Autodesk Inventor part; units mm, degrees
ref_plane "YZ Plane" through (0, 0, 0) normal (1, 0, 0) x (0, 1, 0)
ref_plane "XZ Plane" through (0, 0, 0) normal (0, 1, 0) x (-1, 0, 0)
ref_plane "XY Plane" through (0, 0, 0) normal (0, 0, 1) x (1, 0, 0)
sketch "Sketch1" plane through (0, 0, 0) normal (0, 1, 0) x (-1, 0, 0)
  line L0 (-15, 15) -> (15, 15)
  line L1 (15, 15) -> (15, -15)
  line L2 (15, -15) -> (-15, -15)
  line L3 (-15, -15) -> (-15, 15)
  line L4 (-15, 15) -> (15, -15) construction
  line L5 (15, 15) -> (-15, -15) construction
  circle A0 centre (0, 0) radius 3
  dimension "d0" = 30
  dimension "d1" = 30
  dimension "d2" = 6
extrude "Extrusion1" add sketch "Sketch1" along normal blind 35
The listing builds one solid part. Answer for the finished solid, in the listing's coordinates (mm). Give positions to 0.01 mm unless a question says otherwise; leave off trailing zeros. Order: outer loops, then holes, each group sorted by start corner. A loop starts at its lowest first (then second) coordinate and runs counter-clockwise, first axis right, second up. Notation, with made-up numbers: (45.25, -32.75) -> (66.25, -32.75) arc R27 cw to (66.25, -8.75) -> close; hole circle Ø10 at (46, -31). An arc over 180 degrees is marked (long way). Put each result on its own line as item: value.
Item 1: For a pull along Z with two mould halves and no side action, classify faces 1 (the face through (0, 17, 15)), 2 (the face through (3, 17, 0)), 3 (the face through (0, 17, -15)), 4 (the face through (4, 35, 0)) as released by +Z, released by -Z, zero draft, split by the parting line, or undercut.
Established:
face 1: released by +Z
face 2: undercut
face 3: released by -Z
face 4: zero draft
Item 2: Straight lines are drawn through the part: line 1 (Z direction, x = 0, y = 13); line 2 (X direction, y = 13.5, z = -2); line 3 (X direction, y = 11.5, z = -2.5). For each, find the intervals that lie inside material, in ascending order.
Established:
line 1: z = -15 to -3, 3 to 15
line 2: x = -15 to -2.24, 2.24 to 15
line 3: x = -15 to -1.66, 1.66 to 15
Item 3: A cutting plane is placed at C-C on y = 19. Give the vertices of the cut face in (x, z).
Established:
outline: (-15, -15) -> (15, -15) -> (15, 15) -> (-15, 15) -> close; hole circle Ø6 at (0, 0)
Item 4: A cutting plane is placed at B-B on x = 0. Give the vertices of the cut face in (y, z).
Established:
outline: (0, -15) -> (35, -15) -> (35, -3) -> (0, -3) -> close; (0, 3) -> (35, 3) -> (35, 15) -> (0, 15) -> close
Item 5: A cutting plane is placed at A-A on z = 0. Give the vertices of the cut face in (x, y), plus the area to 3 significant figures.
Established:
outline: (-15, 0) -> (-3, 0) -> (-3, 35) -> (-15, 35) -> close; (3, 0) -> (15, 0) -> (15, 35) -> (3, 35) -> close
area: 840 mm^2
